Geometry check sheet. Reference: the model listing, model coordinates, mm. Give positions to 0.01 mm unless a question says otherwise; leave off trailing zeros. Loops run counter-clockwise (first coordinate to the right, second up) from the corner with the lowest first, then second, coordinate; pieces in that order, holes last. Notation, with made-up numbers: (72, 63) - (122, 63) arc R13 ccw to (122, 82) - close; hole circle Ø6 at (30.5, -35.75). An arc over 180 degrees is marked (long way). Write item = value, one per line. Start each with the question number.
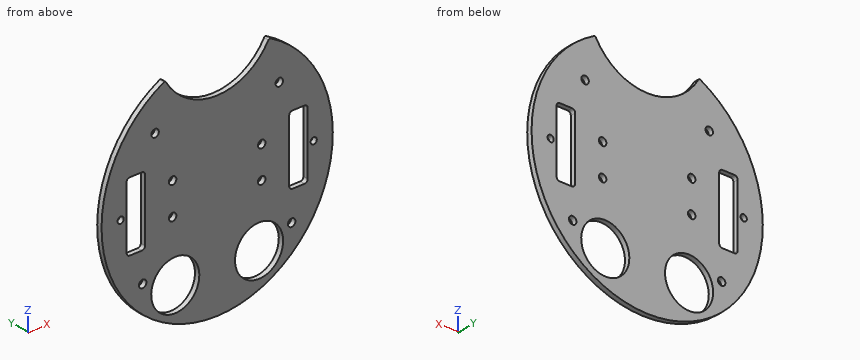
from build123d import *

# Parameters (mm, degrees)
BOSS_EXTRUDE1_DEPTH = 3.2
SKETCH2_W           = 10.76
SKETCH2_H           = 41.868700306
CUT_EXTRUDE1_DEPTH  = 106.40749499
SKETCH3_R           = 2
SKETCH3_R_2         = 2.4
CUT_EXTRUDE2_DEPTH  = 106.40749499
SKETCH4_R           = 15
CUT_EXTRUDE3_DEPTH  = 106.40749499
CUT_EXTRUDE4_DEPTH  = 106.40749499
SKETCH6_R           = 2.4
CUT_EXTRUDE5_DEPTH  = 106.40749499
SKETCH8_R           = 15.5
CUT_EXTRUDE6_DEPTH  = 106.40749499


with BuildPart() as part:
    # Sketch1 → Boss-Extrude1 (new body)
    with BuildSketch(Plane(origin=(0, 0, 0), x_dir=(1, 0, 0), z_dir=(0, 1, 0))):
        with BuildLine():
            ThreePointArc((34.36030176, -66.103098739), (0, 74.5), (-34.36030176, -66.103098739))
            ThreePointArc((-34.36030176, -66.103098739), (-33.621222066, -66.176428208), (-33.035418582, -65.71986465))
            ThreePointArc((-33.035418582, -65.71986465), (0, -46.75), (33.035418582, -65.71986465))
            ThreePointArc((33.035418582, -65.71986465), (33.621222066, -66.176428208), (34.36030176, -66.103098739))
        make_face()
    extrude(amount=BOSS_EXTRUDE1_DEPTH)

    # Sketch2 → Cut-Extrude1 (cut, through all)
    with BuildSketch(Plane(origin=(0, 3.2, 0), x_dir=(1, 0, 0), z_dir=(0, 1, 0))):
        with Locations((-52.39, 0)):
            Rectangle(SKETCH2_W, SKETCH2_H)
        with Locations((52.39, 0)):
            Rectangle(SKETCH2_W, SKETCH2_H)
    extrude(amount=-CUT_EXTRUDE1_DEPTH, mode=Mode.SUBTRACT)

    # Sketch3 → Cut-Extrude2 (cut, through all)
    with BuildSketch(Plane.XZ):
        with Locations(Location((-62.2, 0, 0), (0, 0, 270))):
            Circle(SKETCH3_R)
        with Locations(Location((-28.700738686, 10, 0), (0, 0, 270))):
            Circle(SKETCH3_R_2)
        with Locations(Location((-28.700738686, -10, 0), (0, 0, 270))):
            Circle(SKETCH3_R_2)
        with Locations(Location((28.700738686, -10, 0), (0, 0, 90))):
            Circle(SKETCH3_R_2)
        with Locations(Location((28.700738686, 10, 0), (0, 0, 90))):
            Circle(SKETCH3_R_2)
        with Locations(Location((62.2, 0, 0), (0, 0, 90))):
            Circle(SKETCH3_R)
    extrude(amount=-CUT_EXTRUDE2_DEPTH, mode=Mode.SUBTRACT)

    # Sketch4 → Cut-Extrude3 (cut, through all)
    with BuildSketch(Plane(origin=(0, 3.2, 0), x_dir=(1, 0, 0), z_dir=(0, 1, 0))):
        with Locations(Location((-27, 48, 0), (0, 0, 270))):
            Circle(SKETCH4_R)
        with Locations(Location((27, 48, 0), (0, 0, 90))):
            Circle(SKETCH4_R)
    extrude(amount=-CUT_EXTRUDE3_DEPTH, mode=Mode.SUBTRACT)

    # Sketch5 → Cut-Extrude4 (cut, through all)
    with BuildSketch(Plane(origin=(0, 3.2, 0), x_dir=(1, 0, 0), z_dir=(0, 1, 0))):
        with BuildLine():
            Line((-56.355786438, 21.520136591), (-48.424213562, 21.520136591))
            ThreePointArc((-48.424213562, 21.520136591), (-47.01, 20.934350153), (-46.424213562, 19.520136591))
            Line((-46.424213562, 19.520136591), (-46.424213562, -19.520136591))
            ThreePointArc((-46.424213562, -19.520136591), (-47.01, -20.934350153), (-48.424213562, -21.520136591))
            Line((-48.424213562, -21.520136591), (-56.355786438, -21.520136591))
            ThreePointArc((-56.355786438, -21.520136591), (-57.77, -20.934350153), (-58.355786438, -19.520136591))
            Line((-58.355786438, -19.520136591), (-58.355786438, 19.520136591))
            ThreePointArc((-58.355786438, 19.520136591), (-57.77, 20.934350153), (-56.355786438, 21.520136591))
        make_face()
        with BuildLine():
            Line((46.424213562, 19.520136591), (46.424213562, -19.520136591))
            ThreePointArc((46.424213562, -19.520136591), (47.01, -20.934350153), (48.424213562, -21.520136591))
            Line((48.424213562, -21.520136591), (56.355786438, -21.520136591))
            ThreePointArc((56.355786438, -21.520136591), (57.77, -20.934350153), (58.355786438, -19.520136591))
            Line((58.355786438, -19.520136591), (58.355786438, 19.520136591))
            ThreePointArc((58.355786438, 19.520136591), (57.77, 20.934350153), (56.355786438, 21.520136591))
            Line((56.355786438, 21.520136591), (48.424213562, 21.520136591))
            ThreePointArc((48.424213562, 21.520136591), (47.01, 20.934350153), (46.424213562, 19.520136591))
        make_face()
    extrude(amount=-CUT_EXTRUDE4_DEPTH, mode=Mode.SUBTRACT)

    # Sketch6 → Cut-Extrude5 (cut, through all)
    with BuildSketch(Plane(origin=(0, 3.2, 0), x_dir=(1, 0, 0), z_dir=(0, 1, 0))):
        with Locations(Location((48, 40, 0), (0, 0, 270))):
            Circle(SKETCH6_R)
        with Locations(Location((-40, -40, 0), (0, 0, 270))):
            Circle(SKETCH6_R)
        with Locations(Location((40, -40, 0), (0, 0, 90))):
            Circle(SKETCH6_R)
        with Locations(Location((-48, 40, 0), (0, 0, 90))):
            Circle(SKETCH6_R)
    extrude(amount=-CUT_EXTRUDE5_DEPTH, mode=Mode.SUBTRACT)

    # Sketch8 → Cut-Extrude6 (cut, through all)
    with BuildSketch(Plane(origin=(0, 3.2, 0), x_dir=(1, 0, 0), z_dir=(0, 1, 0))):
        with Locations(Location((-27, 48, 0), (0, 0, 270))):
            Circle(SKETCH8_R)
        with Locations(Location((27, 48, 0), (0, 0, 270))):
            Circle(SKETCH8_R)
    extrude(amount=-CUT_EXTRUDE6_DEPTH, mode=Mode.SUBTRACT)


solid = part.part
1) Cross-section at C-C on x = -40. Enter the section's corners in (y, z), and give its area (3 significant figures).
2) Gauge pin test, flat ends, axial feed: P1, Ø1, axis at x = 53.5, y = 1.5, coming from the -Z side; P2, Ø1, axis at y = 1, z = 4, coming from the +X side; P3, Ø1, axis at x = -15.5, y = 1.5, coming from the -Z side. Record the tip position at first contact, or that the pin passes through.
3) Material ranges on line 1 along X through (y, z) = (2.45, 0); line 2 along X through (y, z) = (2.35, -40); line 3 along X through (y, z) = (2.3, -62), recorded low to high.
4) Cross-section at D-D on y = 1.9. Give the number of separate pieces and of enclosed holes in the cut face, and give its area (3 significant figures).
5) Cross-section at B-B on x = -14.5. Enter the section's corners in (y, z), and give its area (3 significant figures).
6) Cross-section at A-A on z = -51.5. Enter the section's corners in (x, y), and give its area (3 significant figures).
Checked values:
q1.outline = (0, -62.85) - (3.2, -62.85) - (3.2, -56.44) - (0, -56.44) - close; (0, -39.56) - (3.2, -39.56) - (3.2, 37.6) - (0, 37.6) - close; (0, 42.4) - (3.2, 42.4) - (3.2, 62.85) - (0, 62.85) - close
q1.area = 333 mm²
q2.P1 = -52.36
q2.P2 = 74.42
q2.P3 = -72.97
q3.line_1 = -74.5 to -64.2, -60.2 to -58.36, -46.42 to 46.42, 58.36 to 60.2, 64.2 to 74.5
q3.line_2 = -62.85 to -50.4, -45.6 to -40.28, -13.72 to 13.72, 40.28 to 45.6, 50.4 to 62.85
q3.line_3 = -41.31 to -33.65, -20.35 to 20.35, 33.65 to 41.31
q4.separate_pieces = 1
q4.enclosed_holes = 14
q4.area = 13,400 mm²
q5.outline = (0, -73.08) - (3.2, -73.08) - (3.2, -57.17) - (0, -57.17) - close; (0, -38.83) - (3.2, -38.83) - (3.2, 49.6) - (0, 49.6) - close
q5.area = 334 mm²
q6.outline = (-53.83, 0) - (-42.1, 0) - (-42.1, 3.2) - (-53.83, 3.2) - close; (-11.9, 0) - (11.9, 0) - (11.9, 3.2) - (-11.9, 3.2) - close; (42.1, 0) - (53.83, 0) - (53.83, 3.2) - (42.1, 3.2) - close
q6.area = 151 mm²
